Geometry: final body of the model. Coordinates: model frame, mm. Give positions to 0.01 mm unless a question says otherwise; leave off trailing zeros. Order: outer loops, then holes, each group sorted by start corner. A loop starts at its lowest first (then second) coordinate and runs counter-clockwise, first axis right, second up. Notation, with made-up numbers: (24, 29.25) -> (53, 29.25) arc R13 cw to (53, 44.25) -> close; hole circle Ø1 at (78.25, 59). An arc over 180 degrees is marked (long way). Write item = value, one per line.
```python
from build123d import *

# Parameters (mm, degrees)
SKETCH1_W               = 50.8
SKETCH1_H               = 5.08
SOCKET_BODY_DEPTH       = 8.5
SOCKET_HOLES_DEPTH      = 81.873800455
SOCKET_HOLES_DEPTH_BACK = 81.873800455
SKETCH2_W               = 1
SKETCH2_H               = 1


with BuildPart() as part:
    # Sketch1 → Socket_Body (new body)
    with BuildSketch(Plane.XY.offset(4.1)):
        with Locations((32.5, 52.5)):
            Rectangle(SKETCH1_W, SKETCH1_H)
    extrude(amount=SOCKET_BODY_DEPTH)

    # Sketch2 → Socket_Holes (cut, two sides: drawn at the far end of the back side and taken through both)
    with BuildSketch(Plane.XY.offset(-SOCKET_HOLES_DEPTH_BACK)):
        with Locations((8.37, 51.23)):
            Rectangle(SKETCH2_W, SKETCH2_H)
        with Locations((8.37, 53.77)):
            Rectangle(SKETCH2_W, SKETCH2_H)
        with Locations((10.91, 51.23)):
            Rectangle(SKETCH2_W, SKETCH2_H)
        with Locations((10.91, 53.77)):
            Rectangle(SKETCH2_W, SKETCH2_H)
        with Locations((13.45, 51.23)):
            Rectangle(SKETCH2_W, SKETCH2_H)
        with Locations((13.45, 53.77)):
            Rectangle(SKETCH2_W, SKETCH2_H)
        with Locations((15.99, 51.23)):
            Rectangle(SKETCH2_W, SKETCH2_H)
        with Locations((15.99, 53.77)):
            Rectangle(SKETCH2_W, SKETCH2_H)
        with Locations((18.53, 51.23)):
            Rectangle(SKETCH2_W, SKETCH2_H)
        with Locations((18.53, 53.77)):
            Rectangle(SKETCH2_W, SKETCH2_H)
        with Locations((21.07, 51.23)):
            Rectangle(SKETCH2_W, SKETCH2_H)
        with Locations((21.07, 53.77)):
            Rectangle(SKETCH2_W, SKETCH2_H)
        with Locations((23.61, 51.23)):
            Rectangle(SKETCH2_W, SKETCH2_H)
        with Locations((23.61, 53.77)):
            Rectangle(SKETCH2_W, SKETCH2_H)
        with Locations((26.15, 51.23)):
            Rectangle(SKETCH2_W, SKETCH2_H)
        with Locations((26.15, 53.77)):
            Rectangle(SKETCH2_W, SKETCH2_H)
        with Locations((28.69, 51.23)):
            Rectangle(SKETCH2_W, SKETCH2_H)
        with Locations((28.69, 53.77)):
            Rectangle(SKETCH2_W, SKETCH2_H)
        with Locations((31.23, 51.23)):
            Rectangle(SKETCH2_W, SKETCH2_H)
        with Locations((31.23, 53.77)):
            Rectangle(SKETCH2_W, SKETCH2_H)
        with Locations((33.77, 51.23)):
            Rectangle(SKETCH2_W, SKETCH2_H)
        with Locations((33.77, 53.77)):
            Rectangle(SKETCH2_W, SKETCH2_H)
        with Locations((36.31, 51.23)):
            Rectangle(SKETCH2_W, SKETCH2_H)
        with Locations((36.31, 53.77)):
            Rectangle(SKETCH2_W, SKETCH2_H)
        with Locations((38.85, 51.23)):
            Rectangle(SKETCH2_W, SKETCH2_H)
        with Locations((38.85, 53.77)):
            Rectangle(SKETCH2_W, SKETCH2_H)
        with Locations((41.39, 51.23)):
            Rectangle(SKETCH2_W, SKETCH2_H)
        with Locations((41.39, 53.77)):
            Rectangle(SKETCH2_W, SKETCH2_H)
        with Locations((43.93, 51.23)):
            Rectangle(SKETCH2_W, SKETCH2_H)
        with Locations((43.93, 53.77)):
            Rectangle(SKETCH2_W, SKETCH2_H)
        with Locations((46.47, 51.23)):
            Rectangle(SKETCH2_W, SKETCH2_H)
        with Locations((46.47, 53.77)):
            Rectangle(SKETCH2_W, SKETCH2_H)
        with Locations((49.01, 51.23)):
            Rectangle(SKETCH2_W, SKETCH2_H)
        with Locations((49.01, 53.77)):
            Rectangle(SKETCH2_W, SKETCH2_H)
        with Locations((51.55, 51.23)):
            Rectangle(SKETCH2_W, SKETCH2_H)
        with Locations((51.55, 53.77)):
            Rectangle(SKETCH2_W, SKETCH2_H)
        with Locations((54.09, 51.23)):
            Rectangle(SKETCH2_W, SKETCH2_H)
        with Locations((54.09, 53.77)):
            Rectangle(SKETCH2_W, SKETCH2_H)
        with Locations((56.63, 51.23)):
            Rectangle(SKETCH2_W, SKETCH2_H)
        with Locations((56.63, 53.77)):
            Rectangle(SKETCH2_W, SKETCH2_H)
    extrude(amount=SOCKET_HOLES_DEPTH + SOCKET_HOLES_DEPTH_BACK, mode=Mode.SUBTRACT)


solid = part.part
```
1) Line query: line 1 (Y direction, x = 41.5, z = 10.5). Output: solid intervals per line, ascending. Write a range as from..to.
Check sheet entries:
line_1 = 49.96..50.73, 51.73..53.27, 54.27..55.04
2) Section query B-B (z = 11.75). Count the separate pieces of the cut face and the enclosed holes in it, plus the area to 3 significant figures.
Check sheet entries:
separate_pieces = 1
enclosed_holes = 40
area = 218 mm²
3) Section query A-A (x = 51.5). Output: boundary loops of the cut face in (y, z), plus the area to 3 significant figures.
Check sheet entries:
outline = (49.96, 4.1) -> (50.73, 4.1) -> (50.73, 12.6) -> (49.96, 12.6) -> close; (51.73, 4.1) -> (53.27, 4.1) -> (53.27, 12.6) -> (51.73, 12.6) -> close; (54.27, 4.1) -> (55.04, 4.1) -> (55.04, 12.6) -> (54.27, 12.6) -> close
area = 26.2 mm²
